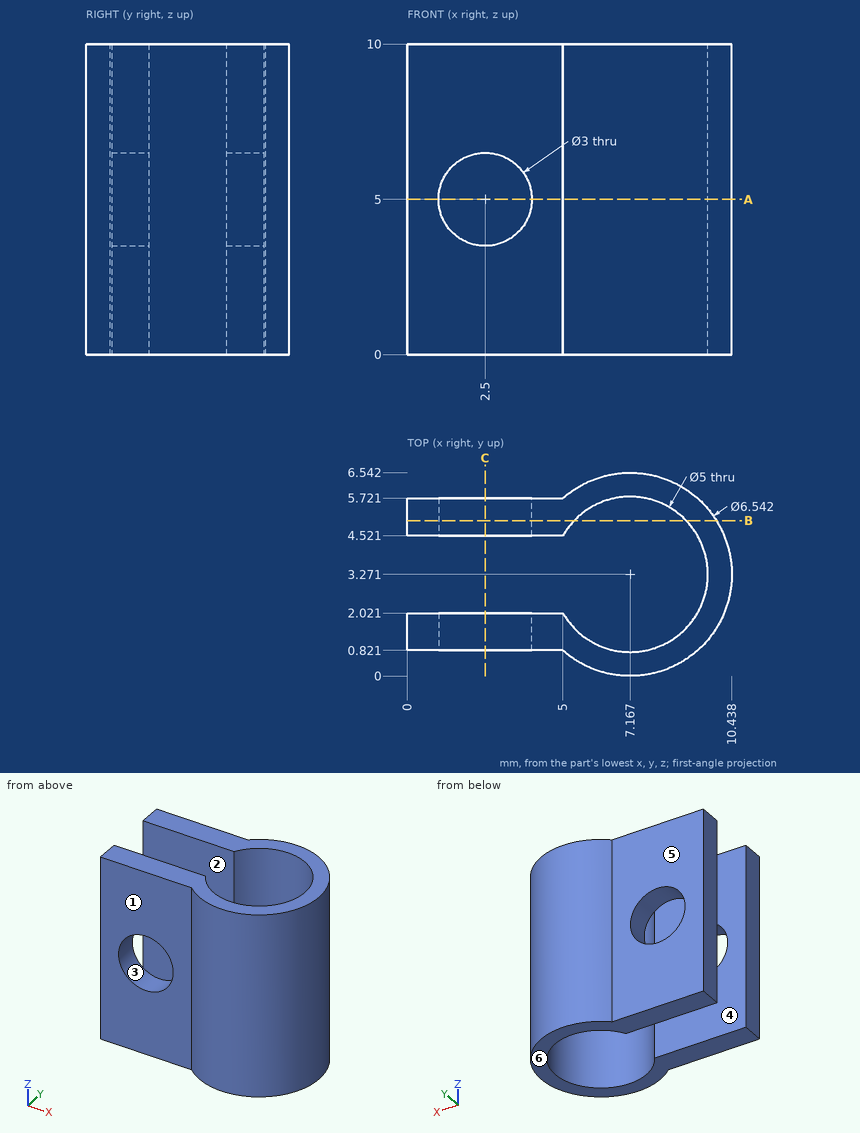
Geometry check sheet. Reference: drawing and pictorial views, mm from the part's lowest x, y, z. A direction names the side the tool comes from. Round coordinates to 2 decimals unless told otherwise and drop trailing zeros. Loops run counter-clockwise (first coordinate to the right, second up) from the corner with the lowest first, then second, coordinate; pieces in that order, holes last. Notation, with made-up numbers: (63, 20.25) - (93, 20.25) arc R19 ccw to (93, 53.25) - close; hole circle Ø8 at (21.5, 30.25). An arc over 180 degrees is marked (long way). Use a Markdown table: item, result. Add a question column.
1. Release check for a two-part mould opening along Y. For the marked faces 4, 5 and 6 record: released by +Y, released by -Y, zero draft, split by the parting line, or undercut.
2. Gauge pin test, flat ends, axial feed: pin 1 (4 mm diameter, centred on x = 2, z = 5, fed in from +Y); pin 2 (3 mm diameter, centred on x = 6.5, z = 1, fed in from +Y); pin 3 (2.5 mm diameter, centred on x = 2, z = 3.5, fed in from -Y). Record the tip position at first contact, or that the pin passes through.
3. Section check A-A, the plane z = 5. Give the number of separate pieces and of enclosed holes in the cut face, plus the area to 3 significant figures.
4. Section check C-C, the plane x = 2.5. Record the boundary of the cut face in (y, z), plus the area to 3 significant figures.
5. Section check B-B, the plane y = 5. Record the boundary of the cut face in (x, z).
6. Thickness scan on probe 1 along Y at (x, z) = (1.5, 7); probe 2 along Z at (x, y) = (2.5, 1.2); probe 3 along X at (y, z) = (1.5, 6.25) (1 decimal). Record the ranges inside material, lowest first. Write a range as [from, to].
7. Access from +Z, -Z, +X, -X, +Y, -Y to the whole of each face (thin tool, end or side, straight path). Record for the marked faces 1, 2 and 3.
Checks:
| question | item | result |
|---|---|---|
| 1 | face 4 | undercut |
| 1 | face 5 | released by +Y |
| 1 | face 6 | zero draft |
| 2 | pin 1 | stops at y = 5.72 |
| 2 | pin 2 | stops at y = 6.54 |
| 2 | pin 3 | stops at y = 0.82 |
| 3 | separate pieces | 3 |
| 3 | enclosed holes | 0 |
| 3 | area | 15.6 mm^2 |
| 4 | outline | (0.82, 0) - (2.02, 0) - (2.02, 3.5) - (0.82, 3.5) - close; (0.82, 6.5) - (2.02, 6.5) - (2.02, 10) - (0.82, 10) - close; (4.52, 0) - (5.72, 0) - (5.72, 3.5) - (4.52, 3.5) - close; (4.52, 6.5) - (5.72, 6.5) - (5.72, 10) - (4.52, 10) - close |
| 4 | area | 16.8 mm^2 |
| 5 | outline | (0, 0) - (5.36, 0) - (5.36, 10) - (0, 10) - close; (8.97, 0) - (9.94, 0) - (9.94, 10) - (8.97, 10) - close; hole circle Ø3 at (2.5, 5) |
| 6 | probe 1 | y = [0.82, 2.02], [4.52, 5.72] |
| 6 | probe 2 | z = [0, 3.5], [6.5, 10] |
| 6 | probe 3 | x = [0, 1.7], [3.3, 5.4], [8.9, 9.9] |
| 7 | face 1 | +Z, -Z, -X, -Y |
| 7 | face 2 | +Z, -Z, -X |
| 7 | face 3 | +Y, -Y |
